For this review, take the finished solid that the model builds, in its own axes (mm). Face numbers are marked on the shaded views. Round coordinates to 2 decimals unless told otherwise and drop trailing zeros. Order: outer loops, then holes, each group sorted by start corner. A loop starts at its lowest first (then second) coordinate and runs counter-clockwise, first axis right, second up.
```python
from build123d import *

# Parameters (mm, degrees)
F0_W        = 118.0765684694
F0_H        = 42.3587011173
F1_DEPTH    = 25.4
F2_T1_DEPTH = 275.8687841416
F3_T1_DEPTH = 417.324487366
F4_R        = 5.08
F5_T1_DEPTH = 59.2305880834
F6_R        = 5.08


# Not quite as in the source:
# - a fillet or chamfer that OpenCascade refuses, or shapes differently, is made with other operations: its cross-section is extruded or revolved along the edge and cut away or added


with BuildPart() as f1:
    # F0 (on Top) → F1 (new body)
    with BuildSketch(Plane.XY):
        with Locations((-49.8337792233, -36.1952199601)):
            Rectangle(F0_W, F0_H)
    extrude(amount=F1_DEPTH)

    # F2: fillet of radius 50.8 on 1 edges, made by hand

    # F2_s2 → F2_t1 (cut)
    with BuildSketch(Plane.XY.offset(-125.2343920708)):
        with BuildLine():
            ThreePointArc((-108.872063458, -15.0158694014), (-91.5793890566, -45.3654069575), (-58.7783066297, -57.3745705187))
            Line((-58.7783066297, -57.3745705187), (-108.872063458, -57.3745705187))
            Line((-108.872063458, -57.3745705187), (-108.872063458, -15.0158694014))
        make_face()
    extrude(amount=F2_T1_DEPTH, mode=Mode.SUBTRACT)

    # F3: chamfer of 76.2 on 1 edges, made by hand

    # F3_s2 → F3_t1 (cut)
    with BuildSketch(Plane.XY.offset(-195.962243683)):
        Polygon((9.2045050114, 18.8254294813), (-66.9954949886, -57.3745705187), (9.2045050114, -57.3745705187), align=None)
    extrude(amount=F3_T1_DEPTH, mode=Mode.SUBTRACT)

    # F4
    f4_edges = [f1.edges().sort_by_distance(p)[0] for p in [
        (-66.417785, -56.79686, 12.7),
    ]]
    fillet(f4_edges, radius=F4_R)

    # F5: fillet of radius 5.08 on 1 edges, made by hand

    # F5_s2 → F5_t1 (cut)
    with BuildSketch(Plane.XY.offset(-16.9152940417)):
        with BuildLine():
            ThreePointArc((-102.4531606824, -15.0158694014), (-106.5420738654, -17.081372929), (-107.3059222438, -21.5982359439))
            ThreePointArc((-107.3059222438, -21.5982359439), (-108.1987038654, -18.3331561934), (-108.872063458, -15.0158694014))
            Line((-108.872063458, -15.0158694014), (-102.4531606824, -15.0158694014))
        make_face()
    extrude(amount=F5_T1_DEPTH, mode=Mode.SUBTRACT)

    # F6
    f6_edges = [f1.edges().sort_by_distance(p)[0] for p in [
        (-44.588616, -34.967691, 0),
        (-66.681498, -56.195765, 0),
        (-92.968648, -44.146642, 0),
        (-106.542074, -17.081373, 0),
        (-63.544977, -15.015869, 0),
    ]]
    fillet(f6_edges, radius=F6_R)


solid = f1.part
```
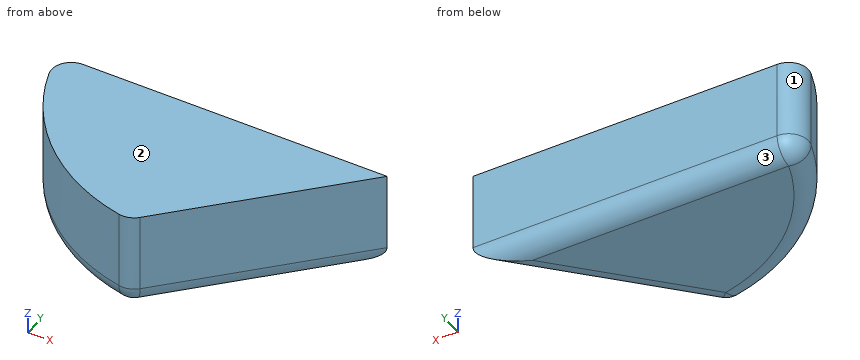
Q1. Clearance check with flat-ended pins moving along their axes: pin 1 (1 mm diameter, centred on y = -20, z = 4, fed in from +X); pin 2 (6 mm diameter, centred on y = -26, z = 20, fed in from -X); pin 3 (5 mm diameter, centred on y = -45, z = 16.5, fed in from +X). State where each tip first meets the part, or that it passes through.
Q2. Wall thickness on line 1 (X direction, y = -21, z = 4.75); line 2 (Y direction, x = -70, z = 5.5); line 3 (Y direction, x = -54, z = 22): over which ranges is each line inside the solid? List them lowest first.
Q3. Take a section at B-B, the plane z = 3. State the section outline as (x, y) points, plus the area to 3 significant figures.
Q4. Mouldability with a two-part tool opening along Z and no side actions: class the marked faces 1, 2 and 3 as +Z half, -Z half, draft (parallel to the pull), parting line (faces both ways), or undercut.
Q5. Take a section at A-A, the plane z = 12.25. State the section outline as (x, y) points.
Working result:
1. pin 1: stops at x = -29.26
1. pin 2: stops at x = -106.85
1. pin 3: stops at x = -52.12
2. line 1: x = -107.44 to -30.64
2. line 2: y = -56.12 to -15.02
2. line 3: y = -44.38 to -15.02
3. outline: (-106.88, -21.47) arc R50.35 ccw to (-69.08, -55.86) arc R4.63 ccw to (-64.86, -54.6) - (-25.71, -15.46) - (-102.45, -15.46) arc R4.63 ccw to start
3. area: 2,050 mm2
4. face 1: draft
4. face 2: +Z half
4. face 3: -Z half
5. outline: (-107.31, -21.6) arc R50.8 ccw to (-69.17, -56.3) arc R5.08 ccw to (-64.54, -54.92) - (-24.64, -15.02) - (-102.45, -15.02) arc R5.08 ccw to start
